```python
from build123d import *

# Parameters (mm, degrees)
F0_W     = 127
F0_H     = 76.2
F1_DEPTH = 63.5
F2_R     = 22.075569
F3_R     = 25.34667
F4_DEPTH = 76.201


with BuildPart() as f1:
    # F0 (on Top) → F1 (new body, symmetric)
    with BuildSketch(Plane.XY):
        Rectangle(F0_W, F0_H)
    extrude(amount=F1_DEPTH, both=True)

    # F2
    f2_edges = [f1.edges().sort_by_distance(p)[0] for p in [
        (-63.5, 0, 63.5),
    ]]
    fillet(f2_edges, radius=F2_R)

    # F3 (on face) → F4 (cut, through all)
    with BuildSketch(Plane(origin=(0, 38.1, 0), x_dir=(-1, 0, 0), z_dir=(0, 1, 0))):
        Circle(F3_R)
    extrude(amount=-F4_DEPTH, mode=Mode.SUBTRACT)


solid = f1.part
```
Input: part model. Units: mm. Frame: model coordinates. Coordinates: 2 decimals unless noted, no trailing zeros. Loops run counter-clockwise (first coordinate to the right, second up) from the corner with the lowest first, then second, coordinate; pieces in that order, holes last. Notation, with made-up numbers: M 61.25,-39 L 69.25,-39 A36 ccw 69.25,-3 Z; hole C 35,-33.75 d5. An arc over 180 degrees is marked long. Use a Markdown table: item, result. Add a question column.
1) Pin query (flat end, axial travel): P1, Ø4, axis at x = -47, y = 18.5, coming from the +Z side. Return the tip coordinate at first contact, or that it passes through.
2) Section C-C, the plane y = 26. Return the cut outline in (x, z), plus the area to 3 significant figures.
3) Section B-B, the plane z = 0. Return the cut outline in (x, y).
4) Draft query along Z for faces 1 (the flat face through (63.5, -1, 1)), 2 (the cylindrical face through (-57.205, 0.533, 56.862)), 3 (the cylindrical face through (5.495, 0.533, -24.744)). Return one class per face: +Z half, -Z half, draft (parallel to the pull), parting line (faces both ways), or undercut.
5) Section A-A, the plane x = 0. Return the cut outline in (y, z), plus the area to 3 significant figures.
6) Line query: L1, parallel to Z at x = 0, y = 20; L2, parallel to Z at x = -13.5, y = 1; L3, parallel to X at y = -25, z = 4.5. Output: solid intervals per line, ascending. Write a range as from..to.
Answer below:
| question | item | result |
|---|---|---|
| 1 | P1 | z = 63.21 |
| 2 | outline | M -63.5,-63.5 L 63.5,-63.5 L 63.5,63.5 L -41.42,63.5 A22.08 ccw -63.5,41.42 Z; hole C 0,0 d50.69 |
| 2 | area | 14,000 mm2 |
| 3 | outline | M -63.5,-38.1 L -25.35,-38.1 L -25.35,38.1 L -63.5,38.1 Z; M 25.35,-38.1 L 63.5,-38.1 L 63.5,38.1 L 25.35,38.1 Z |
| 4 | face 1 | draft |
| 4 | face 2 | +Z half |
| 4 | face 3 | undercut |
| 5 | outline | M -38.1,-63.5 L 38.1,-63.5 L 38.1,-25.35 L -38.1,-25.35 Z; M -38.1,25.35 L 38.1,25.35 L 38.1,63.5 L -38.1,63.5 Z |
| 5 | area | 5,810 mm2 |
| 6 | L1 | -63.5..-25.35, 25.35..63.5 |
| 6 | L2 | -63.5..-21.45, 21.45..63.5 |
| 6 | L3 | -63.5..-24.94, 24.94..63.5 |
